Verification items for this drawing (mm, ordinates from the low corner). Round coordinates to 2 decimals unless told otherwise and drop trailing zeros. Write each loop counter-clockwise with the first axis right and the second up, starting at its lowest first coordinate (ties: lowest second). Pieces come first, ordered by that corner, then holes. Notation, with made-up numbers: (87.5, 16) -> (101.5, 16) arc R10 ccw to (101.5, 34) -> close; hole circle Ø7 at (16.25, -27). An arc over 180 degrees is marked (long way). Return JSON: item names as keys, results as strings. Group by question number.
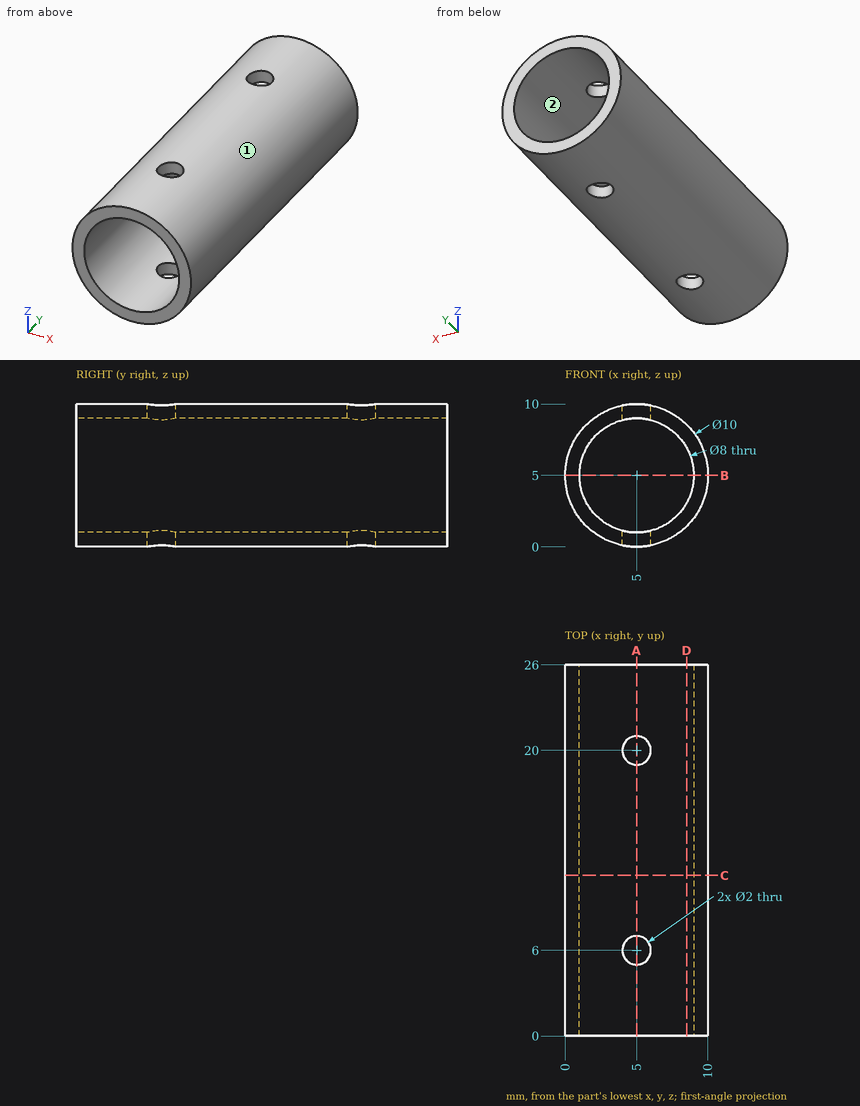
1) Sectioned sample at C-C on y = 11.25. Enter the section's corners in (x, z).
2) Mould release check, pull along X, two halves, no side actions. Record for the marked faces 1 and 2: +X half, -X half, draft (parallel to the pull), parting line (faces both ways), or undercut.
3) Sectioned sample at A-A on x = 5. Enter the section's corners in (y, z).
4) Go/stop test with flat-tipped pins: P1, Ø1.2, axis at x = 5, y = 20, coming from the -Z side; P2, Ø2, axis at y = 7.5, z = 8.5, coming from the +X side; P3, Ø6, axis at y = 11, z = 8.5, coming from the +X side. Record where each tip stops, or that it passes through.
5) Sectioned sample at B-B on z = 5. Enter the section's corners in (x, y), and give its area (3 significant figures).
6) Sectioned sample at D-D on x = 8.5. Enter the section's corners in (y, z), and give its area (3 significant figures).
7) Material ranges on probe 1 along Y at (x, z) = (5, 0.6); probe 2 along Z at (x, y) = (6, 20.5); probe 3 along X at (y, z) = (16.5, 8.25), recorded low to high. Write a range as [from, to].
Evaluation:
{
 "1": {"outline": "circle Ø10 at (5, 5); hole circle Ø8 at (5, 5)"},
 "2": {"face 1": "parting line", "face 2": "undercut"},
 "3": {"outline": "(0, 0) -> (5, 0) -> (5, 1) -> (0, 1) -> close; (0, 9) -> (5, 9) -> (5, 10) -> (0, 10) -> close; (7, 0) -> (19, 0) -> (19, 1) -> (7, 1) -> close; (7, 9) -> (19, 9) -> (19, 10) -> (7, 10) -> close; (21, 0) -> (26, 0) -> (26, 1) -> (21, 1) -> close; (21, 9) -> (26, 9) -> (26, 10) -> (21, 10) -> close"},
 "4": {"P1": "passes through", "P2": "stops at x = 9.33", "P3": "stops at x = 9.97"},
 "5": {"outline": "(0, 0) -> (1, 0) -> (1, 26) -> (0, 26) -> close; (9, 0) -> (10, 0) -> (10, 26) -> (9, 26) -> close", "area": "52.0 mm2"},
 "6": {"outline": "(0, 1.43) -> (26, 1.43) -> (26, 3.06) -> (0, 3.06) -> close; (0, 6.94) -> (26, 6.94) -> (26, 8.57) -> (0, 8.57) -> close", "area": "85.0 mm2"},
 "7": {"probe 1": "y = [0, 5], [7, 19], [21, 26]", "probe 2": "z = [0.1, 1.13], [8.87, 9.9]", "probe 3": "x = [1.2, 2.67], [7.33, 8.8]"}
}
